```python
from build123d import *

# Parameters (mm, degrees)
SKETCH1_R           = 16.5
SKETCH1_R_2         = 1.2
SKETCH1_R_3         = 9.5
SKETCH1_R_4         = 1.55
BOSS_EXTRUDE1_DEPTH = 9
SKETCH2_R           = 3.7
CUT_EXTRUDE1_DEPTH  = 6


with BuildPart() as part:
    # Sketch1 → Boss-Extrude1 (new body)
    with BuildSketch(Plane.XY):
        Circle(SKETCH1_R)
        with Locations((8.980256121, 8.980256121)):
            Circle(SKETCH1_R_2, mode=Mode.SUBTRACT)
        with Locations((8.980256121, -8.980256121)):
            Circle(SKETCH1_R_2, mode=Mode.SUBTRACT)
        with Locations((-8.980256121, -8.980256121)):
            Circle(SKETCH1_R_2, mode=Mode.SUBTRACT)
        with Locations((-8.980256121, 8.980256121)):
            Circle(SKETCH1_R_2, mode=Mode.SUBTRACT)
        Circle(SKETCH1_R_3, mode=Mode.SUBTRACT)
        with Locations((0, 13)):
            Circle(SKETCH1_R_4, mode=Mode.SUBTRACT)
        with Locations((13, 0)):
            Circle(SKETCH1_R_4, mode=Mode.SUBTRACT)
        with Locations((0, -13)):
            Circle(SKETCH1_R_4, mode=Mode.SUBTRACT)
        with Locations((-13, 0)):
            Circle(SKETCH1_R_4, mode=Mode.SUBTRACT)
    extrude(amount=BOSS_EXTRUDE1_DEPTH)

    # Sketch2 → Cut-Extrude1 (cut)
    with BuildSketch(Plane.XY.offset(9)):
        with Locations((0, 13)):
            Circle(SKETCH2_R)
        with Locations((13, 0)):
            Circle(SKETCH2_R)
        with Locations((0, -13)):
            Circle(SKETCH2_R)
        with Locations((-13, 0)):
            Circle(SKETCH2_R)
    extrude(amount=-CUT_EXTRUDE1_DEPTH, mode=Mode.SUBTRACT)


solid = part.part
```
Read the model definition and answer for the solid it produces. Units are mm, in the model's axes. A direction names the side the tool comes from. Give positions to 0.01 mm unless a question says otherwise; leave off trailing zeros. Order: outer loops, then holes, each group sorted by start corner. A loop starts at its lowest first (then second) coordinate and runs counter-clockwise, first axis right, second up.
(1) Find section B-B (z = 4.5). Give the vertices of the cut face in (x, y).
(2) Straight lines are drawn through the part: L1, parallel to Y at x = 0, z = 1.4; L2, parallel to X at y = -2.5, z = 8.25; L3, parallel to Y at x = -2, z = 7.75. For each, find the intervals that lie inside material, in ascending order.
(3) Given pin 1 (3.5 mm diameter, centred on x = 0, y = -13, fed in from -Z); pin 2 (2.5 mm diameter, centred on x = 0, y = 13, fed in from +Z); pin 3 (4 mm diameter, centred on y = -8, z = 6, fed in from +X); pin 4 (2 mm diameter, centred on x = 1, y = 13, fed in from +Z), each flat-ended and moving along its own axis, determine where each tip first touches the part or whether it passes through.
(4) For faces 1 (the cylindrical face through (-3.692, -12.763, 6.042)), 2 (the cylindrical face through (-10.18, -8.93, 4.44)), determine the directions among +Z, -Z, +X, -X, +Y, -Y from which every point of the face is accessible in a straight line to the end or side of a thin tool.
(5) Find section D-D (y = 4.5). Give the vertices of the cut face in (x, z).
(6) For a pull along X with two mould halves and no side action, classify faces 3 (the cylindrical face through (15.738, 4.956, 4.437)), 4 (the cylindrical face through (-3.7, 12.9, 6)), 5 (the flat face through (-8.84, -10.34, 9)) as released by +X, released by -X, zero draft, split by the parting line, or undercut.
(7) Find section A-A (y = 0). Give the vertices of the cut face in (x, z).
Result sheet:
1. outline: (-16.44, -1.35) arc R16.5 ccw to (-1.35, -16.44) arc R3.7 cw to (-1.02, -9.44) arc R9.5 cw to (-9.44, -1.02) arc R3.7 cw to start; (-16.44, 1.35) arc R3.7 cw to (-9.44, 1.02) arc R9.5 cw to (-1.02, 9.44) arc R3.7 cw to (-1.35, 16.44) arc R16.5 ccw to start; (1.02, -9.44) arc R3.7 cw to (1.35, -16.44) arc R16.5 ccw to (16.44, -1.35) arc R3.7 cw to (9.44, -1.02) arc R9.5 cw to start; (1.02, 9.44) arc R9.5 cw to (9.44, 1.02) arc R3.7 cw to (16.44, 1.35) arc R16.5 ccw to (1.35, 16.44) arc R3.7 cw to start; hole circle Ø2.4 at (-8.98, -8.98); hole circle Ø2.4 at (-8.98, 8.98); hole circle Ø2.4 at (8.98, -8.98); hole circle Ø2.4 at (8.98, 8.98)
2. L1: y = -16.5 to -14.55, -11.45 to -9.5, 9.5 to 11.45, 14.55 to 16.5
2. L2: x = -16.31 to -15.73, -10.27 to -9.17, 9.17 to 10.27, 15.73 to 16.31
2. L3: y = -16.38 to -16.11, -9.89 to -9.29, 9.29 to 9.89, 16.11 to 16.38
3. pin 1: stops at z = 0
3. pin 2: passes through
3. pin 3: stops at x = 15.37
3. pin 4: stops at z = 3
4. face 1: +Z
4. face 2: +Z, -Z
5. outline: (-15.87, 0) - (-8.37, 0) - (-8.37, 9) - (-15.87, 9) - close; (8.37, 0) - (15.87, 0) - (15.87, 9) - (8.37, 9) - close
6. face 3: split by the parting line
6. face 4: undercut
6. face 5: zero draft
7. outline: (-16.5, 0) - (-14.55, 0) - (-14.55, 3) - (-16.5, 3) - close; (-11.45, 0) - (-9.5, 0) - (-9.5, 3) - (-11.45, 3) - close; (9.5, 0) - (11.45, 0) - (11.45, 3) - (9.5, 3) - close; (14.55, 0) - (16.5, 0) - (16.5, 3) - (14.55, 3) - close
